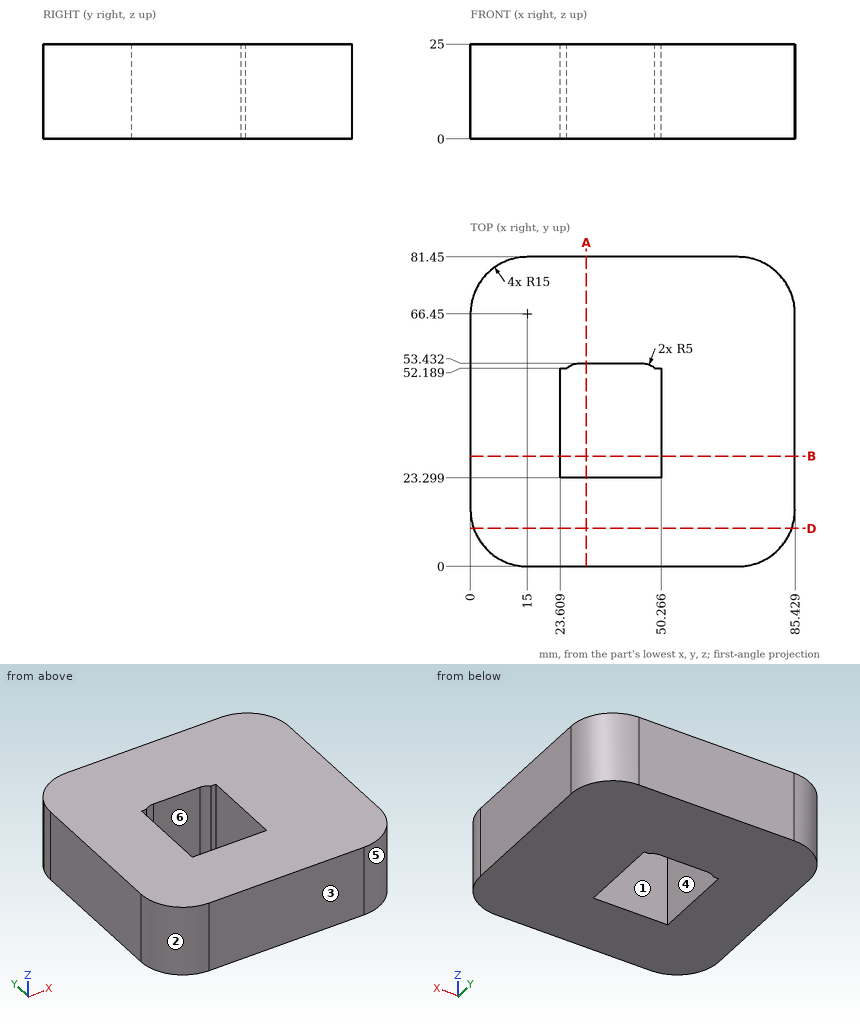
Part print with two shaded views. Sizes in mm from the minimum x, y, z corner. A direction names the side the tool comes from. Round coordinates to 2 decimals unless told otherwise and drop trailing zeros. Write each loop counter-clockwise with the first axis right and the second up, starting at its lowest first coordinate (ties: lowest second). Pieces come first, ordered by that corner, then holes. Notation, with made-up numbers: (28.5, 74.5) - (57.5, 74.5) arc R28 ccw to (57.5, 103.5) - close; hole circle Ø7 at (-4.5, 45.25). An arc over 180 degrees is marked (long way). Use CSV: the item, a comma, the result in double quotes.
Item 1: Slice it at D-D, the plane y = 10. Write the cut outline in (x, z), then the cut area to 3 significant figures.
Results list:
outline,"(0.86, 0) - (84.57, 0) - (84.57, 25) - (0.86, 25) - close"
area,"2,090 mm²"
Item 2: Tool access for the marked faces 1 and 2: list every direction of +Z, -Z, +X, -X, +Y, -Y with a clear straight run to the whole face (end or side of a thin tool).
Results list:
face 1,"+Z, -Z"
face 2,"+Z, -Z, -X, -Y"
Item 3: Pull direction X, two halves, no side cores. Call the marked faces 3, 4, 5 and 6: pulls with the +X half, pulls with the -X half, needs draft (parallel to the pull), parting line crosses it, or undercut.
Results list:
face 3,"needs draft"
face 4,"undercut"
face 5,"pulls with the +X half"
face 6,"undercut"
Item 4: Flat gauge pin, fed straight in: P1, Ø6, axis at x = 55.5, y = 30, coming from the -Z side. Where does the tip first touch, or does it go through?
Results list:
P1,"stops at z = 0"
Item 5: Slice it at B-B, the plane y = 29. Write the cut outline in (x, z), then the cut area to 3 significant figures.
Results list:
outline,"(0, 0) - (23.61, 0) - (23.61, 25) - (0, 25) - close; (50.27, 0) - (85.43, 0) - (85.43, 25) - (50.27, 25) - close"
area,"1,470 mm²"
Item 6: Wall check: L1, parallel to X at y = 49, z = 20; L2, parallel to Y at x = 45, z = 17.25; L3, parallel to X at y = 12, z = 23 (1 decimal). Give the ranges that are in metal, low to high.
Results list:
L1,"x = 0 to 23.61, 50.27 to 85.43"
L2,"y = 0 to 23.3, 53.43 to 81.45"
L3,"x = 0.3 to 85.1"
Item 7: Slice it at A-A, the plane x = 30.5. Write the cut outline in (y, z).
Results list:
outline,"(0, 0) - (23.3, 0) - (23.3, 25) - (0, 25) - close; (53.43, 0) - (81.45, 0) - (81.45, 25) - (53.43, 25) - close"
